Part model, mm, in its own coordinate system. A direction names the side the tool comes from. Coordinates: 2 decimals unless noted, no trailing zeros. Write each loop counter-clockwise with the first axis right and the second up, starting at its lowest first coordinate (ties: lowest second). Pieces come first, ordered by that corner, then holes. Notation, with made-up numbers: (-40, 31.25) - (1, 31.25) arc R38 ccw to (1, 69.25) - close; hole circle Ø10 at (21.25, -31). An arc over 180 degrees is marked (long way). Write each question's results on one line, items separated by ' | '.
Autodesk Inventor part; units mm, degrees
ref_plane "YZ Plane" through (0, 0, 0) normal (1, 0, 0) x (0, 1, 0)
ref_plane "XZ Plane" through (0, 0, 0) normal (0, 1, 0) x (-1, 0, 0)
ref_plane "XY Plane" through (0, 0, 0) normal (0, 0, 1) x (1, 0, 0)
sketch "Sketch1" plane through (0, 0, 0) normal (0, 1, 0) x (-1, 0, 0)
  line L0 (0, 0) -> (-300, 0)
  line L1 (-300, 0) -> (-300, -23.685)
  line L2 (-300, -23.685) -> (0, -23.685)
  line L3 (0, -23.685) -> (0, 0)
  dimension "d0" = 300
  dimension "d1" = 23.685
extrude "Extrusion1" add sketch "Sketch1" along normal blind 6.5
sketch "Sketch2" plane through (0, 6.5, 0) normal (0, 1, 0) x (1, 0, 0)
  line L0 (0, 23.685) -> (0, 0)
  line L1 (21, 19.3425) -> (27, 19.3425)
  line L2 (28, 18.3425) -> (28, 5.3425)
  line L3 (27, 4.3425) -> (21, 4.3425)
  line L4 (20, 5.3425) -> (20, 18.3425)
  arc A0 (21, 19.3425) -> (20, 18.3425) centre (21, 18.3425) ccw
  arc A1 (20, 5.3425) -> (21, 4.3425) centre (21, 5.3425) ccw
  arc A2 (27, 4.3425) -> (28, 5.3425) centre (27, 5.3425) ccw
  arc A3 (28, 18.3425) -> (27, 19.3425) centre (27, 18.3425) ccw
  point P0 (20, 11.8425)
  point P1 (0, 11.8425)
  dimension "d4" = 1
  dimension "d5" = 15
  dimension "d6" = 8
  dimension "d7" = 20
extrude "Extrusion2" cut sketch "Sketch2" against normal through all
pattern_linear "Rectangular Pattern1" count 5 spacing 12 along (1, 0, 0) of "Extrusion2"
properties part number "front_pane_middle"
(1) Wall check: line 1 (X direction, y = 3.5, z = -8.75); line 2 (Z direction, x = 50, y = 1.5) (1 decimal); line 3 (Z direction, x = 56.5, y = 3.5) (3 decimals). Give the ranges that are in metal, low to high. Write a range as from..to.
Return value:
line 1: x = 0..20, 28..32, 40..44, 52..56, 64..68, 76..300 | line 2: z = -23.7..-19.3, -4.3..0 | line 3: z = -23.685..-19.209, -4.476..0
(2) Two-plate mould, pull along Z, no slides. Class faces 1 (the flat face through (32, 3, -12)), 2 (the flat face through (300, 3, -12)), 3 (the flat face through (152, 3, -23.685)): released by +Z, released by -Z, zero draft, split by the parting line, or undercut.
Return value:
face 1: undercut | face 2: zero draft | face 3: released by -Z
(3) Saw through at B-B on y = 3. Count the separate pieces of the cut face and the enclosed holes in it, then the cut area to 3 significant figures.
Return value:
separate pieces: 1 | enclosed holes: 5 | area: 6,510 mm^2
(4) Saw through at A-A on z = -14.5. Write the cut outline in (x, y), then the cut area to 3 significant figures.
Return value:
outline: (0, 0) - (20, 0) - (20, 6.5) - (0, 6.5) - close; (28, 0) - (32, 0) - (32, 6.5) - (28, 6.5) - close; (40, 0) - (44, 0) - (44, 6.5) - (40, 6.5) - close; (52, 0) - (56, 0) - (56, 6.5) - (52, 6.5) - close; (64, 0) - (68, 0) - (68, 6.5) - (64, 6.5) - close; (76, 0) - (300, 0) - (300, 6.5) - (76, 6.5) - close | area: 1,690 mm^2
(5) 3-axis set-ups, long thin cutter, end or side, ignore diameter. For faces 4 (the flat face through (60, 3, -19.342)), 5 (the flat face through (152, 6.5, -12)): which of +Z, -Z, +X, -X, +Y, -Y reach the whole face in a straight line?
Return value:
face 4: +Y, -Y | face 5: +Z, -Z, +X, -X, +Y
